Could you check a few things on this model? Use its own coordinates, in mm. Coordinates: 2 decimals unless noted, no trailing zeros. Write each loop counter-clockwise with the first axis right and the second up, starting at its lowest first coordinate (ties: lowest second). Pieces come first, ordered by that corner, then holes. Notation, with made-up numbers: M 47,-31.75 L 53,-31.75 A19 ccw 53,-15.75 Z; hole C -21.75,-3.75 d2. An arc over 180 degrees is marked long. Answer as CSV lines item,"result". Start each with the question number.
Item 1: Suppose I cut it at B-B, the plane z = 13.5. Write out the boundary of the cut face in (x, y), and give its area (3 significant figures).
Item 2: If I drill on line 1 along Z through (x, y) = (9, 20.5); line 2 along X through (y, z) = (53, 71); line 3 along Y through (x, z) = (38, 124), over which ranges is the centre line in solid material (lowest first)? Write a range as [from, to].
Item 3: Suppose I cut it at A-A, the plane y = 56. Write out the boundary of the cut face in (x, z).
```python
from build123d import *

# Parameters (mm, degrees)
ESQUISSE1_W        = 45
ESQUISSE1_H        = 60
BOSS_EXTRU_1_DEPTH = 170
CONG_1_R           = 10


with BuildPart() as part:
    # Esquisse1 → Boss.-Extru.1 (new body)
    with BuildSketch(Plane.XY):
        with Locations((22.5, 30)):
            Rectangle(ESQUISSE1_W, ESQUISSE1_H)
    extrude(amount=BOSS_EXTRU_1_DEPTH)

    # Congé1
    cong_1_edges = [part.edges().sort_by_distance(p)[0] for p in [
        (45, 30, 170),
        (22.5, 60, 170),
        (0, 30, 170),
        (22.5, 60, 0),
        (45, 30, 0),
        (22.5, 0, 0),
        (0, 30, 0),
        (22.5, 0, 170),
        (0, 60, 85),
        (45, 60, 85),
        (45, 0, 85),
        (0, 0, 85),
    ]]
    fillet(cong_1_edges, radius=CONG_1_R)


solid = part.part
```
Ans:
1,outline,"M 0,10 A10 ccw 10,0 L 35,0 A10 ccw 45,10 L 45,50 A10 ccw 35,60 L 10,60 A10 ccw 0,50 Z"
1,area,"2,610 mm^2"
2,line 1,"z = [0.05, 169.95]"
2,line 2,"x = [0.46, 44.54]"
2,line 3,"y = [0.46, 59.54]"
3,outline,"M 2,10 A8 ccw 10,2 L 35,2 A8 ccw 43,10 L 43,160 A8 ccw 35,168 L 10,168 A8 ccw 2,160 Z"
